from build123d import *

# Parameters (mm, degrees)
F3_DEPTH = 25.4
F0_W     = 12.7
F0_H     = 12.7
F4_DEPTH = 25.4
F5_DEPTH = 25.4


with BuildPart() as f3:
    # F1 (on Top) → F3 (new body)
    with BuildSketch(Plane.XY):
        Polygon((19.05, 25.4), (0, 25.4), (25.4, 0), (38.1, 0), (38.1, 6.35), align=None)
    extrude(amount=F3_DEPTH)

    # F0 (on Front) → F4 (join)
    with BuildSketch(Plane.XZ):
        with Locations((31.75, 19.05)):
            Rectangle(F0_W, F0_H)
    extrude(amount=-F4_DEPTH)

    # F2 (on Right) → F5 (join)
    with BuildSketch(Plane.YZ):
        Polygon((0, 12.7), (0, 0), (25.4, 0), (25.4, 25.4), (6.35, 25.4), (6.35, 12.7), align=None)
    extrude(amount=F5_DEPTH)


solid = f3.part
Geometry: final body of the model. Coordinates: model frame, mm. A direction names the side the tool comes from. Give positions to 0.01 mm unless a question says otherwise; leave off trailing zeros. Write each loop counter-clockwise with the first axis right and the second up, starting at its lowest first coordinate (ties: lowest second). Pieces come first, ordered by that corner, then holes.
(1) Ray query, line 1 (Y direction, x = 9.5, z = 20); line 2 (Z direction, x = 28, y = 21.25); line 3 (X direction, y = 20, z = 11.5). Return the intervals inside material, ascending.
(2) First-contact query: P1, Ø7, axis at y = 21, z = 5.5, coming from the +X side; P2, Ø5, axis at y = 14, z = 3, coming from the +X side; P3, Ø1.5, axis at x = 7.5, z = 4.5, coming from the -Y side; P4, Ø6.5, axis at x = 32, y = 19, coming from the -Z side. Flat tips, straight axial feed; report the tip coordinate or a pass-through.
(3) Cut plane A-A, the plane x = 34.5. Return loops of the section in (y, z), then the cut area to 3 significant figures.
(4) Access query for faces 1 (the flat face through (33, 18, 12.7)), 2 (the flat face through (38.1, 10, 18)), 3 (the flat face through (9, 6.35, 19)). Directions: +Z, -Z, +X, -X, +Y, -Y. A direction counts if a zero-diameter tool reaches every point of the face in a straight line with its end or side. Return the directions, or none.
(5) Cut plane B-B, the plane y = 8.5. Return loops of the section in (x, z).
Values follow:
1. line 1: y = 6.35 to 25.4
1. line 2: z = 12.7 to 25.4
1. line 3: x = 0 to 25.4
2. P1: stops at x = 26.95
2. P2: stops at x = 32.95
2. P3: stops at y = 0
2. P4: stops at z = 12.7
3. outline: (0, 0) - (9.95, 0) - (9.95, 12.7) - (25.4, 12.7) - (25.4, 25.4) - (0, 25.4) - close
3. area: 449 mm2
4. face 1: -Z, +X, +Y
4. face 2: +Z, -Z, +X, +Y, -Y
4. face 3: +Z, -X, -Y
5. outline: (0, 0) - (35.95, 0) - (35.95, 12.7) - (38.1, 12.7) - (38.1, 25.4) - (0, 25.4) - close
